```python
from build123d import *

# Parameters (mm, degrees)
F0_W           = 152.4
F0_H           = 105.41
F1_DEPTH       = 12.7
F3_D           = 6.35
F3_CBORE_D     = 9.525
F3_CBORE_DEPTH = 6.35
F4_W           = 101.6
F4_H           = 105.41
F5_DEPTH       = 101.6
F6_R           = 25.4
F7_R           = 6.35
F8_R           = 39.6875
F9_DEPTH       = 105.411
F10_R          = 2.286
F11_SIZE       = 0.7874


with BuildPart() as f1:
    # F0 (on Front) → F1 (new body)
    with BuildSketch(Plane.XZ):
        with Locations((-76.2, 52.705)):
            Rectangle(F0_W, F0_H)
    extrude(amount=F1_DEPTH)

    # F3 (through all)
    with Locations(Plane.XZ.offset(12.7)):
        with Locations((-9.525, 92.71), (-142.875, 92.71), (-9.525, 12.7), (-142.875, 12.7)):
            CounterBoreHole(F3_D / 2, F3_CBORE_D / 2, F3_CBORE_DEPTH)

    # F4 (on face) → F5 (join)
    with BuildSketch(Plane.XZ.offset(12.7)):
        with Locations((-76.2, 52.705)):
            Rectangle(F4_W, F4_H)
    extrude(amount=F5_DEPTH)

    # F6
    f6_edges = [f1.edges().sort_by_distance(p)[0] for p in [
        (-25.4, -114.3, 52.705),
        (-127, -114.3, 52.705),
    ]]
    fillet(f6_edges, radius=F6_R)

    # F7
    f7_edges = [f1.edges().sort_by_distance(p)[0] for p in [
        (-25.4, -12.7, 52.705),
        (-127, -12.7, 52.705),
    ]]
    fillet(f7_edges, radius=F7_R)

    # F8 (on face) → F9 (cut, through all)
    with BuildSketch(Plane(origin=(0, 0, 0), x_dir=(1, 0, 0), z_dir=(0, 0, -1))):
        with Locations((-76.2, 63.5)):
            Circle(F8_R)
    extrude(amount=-F9_DEPTH, mode=Mode.SUBTRACT)

    # F10
    f10_edges = [f1.edges().sort_by_distance(p)[0] for p in [
        (-142.875, -12.7, 0),
        (-9.525, -12.7, 0),
        (0, -12.7, 52.705),
        (-142.875, -12.7, 105.41),
        (-9.525, -12.7, 105.41),
        (-76.2, 0, 105.41),
        (0, 0, 52.705),
        (-152.4, -12.7, 52.705),
        (-152.4, 0, 52.705),
        (-76.2, 0, 0),
    ]]
    fillet(f10_edges, radius=F10_R)

    # F11
    f11_edges = [f1.edges().sort_by_distance(p)[0] for p in [
        (-115.8875, -63.5, 105.41),
        (-115.8875, -63.5, 0),
    ]]
    chamfer(f11_edges, length=F11_SIZE)


solid = f1.part
```
Check sheet for the modelled part. Datum: model origin and axes. Units: mm. A direction names the side the tool comes from. Give positions to 0.01 mm unless a question says otherwise; leave off trailing zeros. Loops run counter-clockwise (first coordinate to the right, second up) from the corner with the lowest first, then second, coordinate; pieces in that order, holes last. Notation, with made-up numbers: M -28,52 L -17,52 A17 cw -17,78 Z; hole C -16.5,2 d5. An arc over 180 degrees is marked long. Answer in a Markdown table with one row per item.
1) Cross-section at C-C (y = -63.5). Enter the section's corners in (x, z), plus the area to 3 significant figures.
Solutions:
| item | result |
|---|---|
| outline | M -127,2.29 A2.29 ccw -124.71,0 L -116.67,0 L -115.89,0.79 L -115.89,104.62 L -116.67,105.41 L -124.71,105.41 A2.29 ccw -127,103.12 Z; M -36.51,0.79 L -35.73,0 L -27.69,0 A2.29 ccw -25.4,2.29 L -25.4,103.12 A2.29 ccw -27.69,105.41 L -35.73,105.41 L -36.51,104.62 Z |
| area | 2,340 mm^2 |
2) Depth check by flat-ended pin: pin 1 (10.5 mm diameter, centred on x = -140.5, z = 14, fed in from -Y); pin 2 (5 mm diameter, centred on x = -9.5, z = 11, fed in from -Y); pin 3 (5 mm diameter, centred on y = -18.5, z = 29.5, fed in from +X). Enter the tip coordinate at first touch or a pass-through.
Solutions:
| item | result |
|---|---|
| pin 1 | stops at y = -12.7 |
| pin 2 | stops at y = -6.35 |
| pin 3 | stops at x = -24.62 |
3) Cross-section at A-A (z = 92.71). Count the separate pieces of the cut face and the enclosed holes in it, plus the area to 3 significant figures.
Solutions:
| item | result |
|---|---|
| separate pieces | 3 |
| enclosed holes | 1 |
| area | 6,840 mm^2 |
4) Mould release check, pull along X, two halves, no side actions. Record for faces 4 (the face through (-119.76, -106.66, 53.41)), 5 (the face through (-6, -6.35, 12)), 6 (the face through (-23.59, -14.61, 53.41)), 7 (the face through (-142, -12.7, 53)): released by +X, released by -X, zero draft, split by the parting line, or undercut.
Solutions:
| item | result |
|---|---|
| face 4 | released by -X |
| face 5 | undercut |
| face 6 | released by +X |
| face 7 | zero draft |
5) Thickness scan on line 1 (X direction, y = -63, z = 31); line 2 (X direction, y = -10, z = 12); line 3 (Y direction, x = -76.2, z = 69). Record the ranges inside material, lowest first.
Solutions:
| item | result |
|---|---|
| line 1 | x = -127 to -115.88, -36.52 to -25.4 |
| line 2 | x = -152.4 to -147.59, -138.16 to -14.24, -4.81 to 0 |
| line 3 | y = -114.3 to -103.19, -23.81 to 0 |
6) Cross-section at B-B (x = -76.2). Enter the section's corners in (y, z).
Solutions:
| item | result |
|---|---|
| outline | M -114.3,2.29 A2.29 ccw -112.01,0 L -103.97,0 L -103.19,0.79 L -103.19,104.62 L -103.97,105.41 L -112.01,105.41 A2.29 ccw -114.3,103.12 Z; M -23.81,0.79 L -23.03,0 L -2.29,0 A2.29 ccw 0,2.29 L 0,103.12 A2.29 ccw -2.29,105.41 L -23.03,105.41 L -23.81,104.62 Z |
7) Tool access check on faces 1 (the face through (-143.91, -9.57, 88.06)), 2 (the face through (-11, -12.7, 53)), 3 (the face through (-142.462, -3.131, 95.858)). Record the directions out of +Z, -Z, +X, -X, +Y, -Y that give a thin tool (end or side, any length) a straight path to the whole face; none if there is none.
Solutions:
| item | result |
|---|---|
| face 1 | -Y |
| face 2 | +Z, -Z, +X, -Y |
| face 3 | +Y, -Y |
